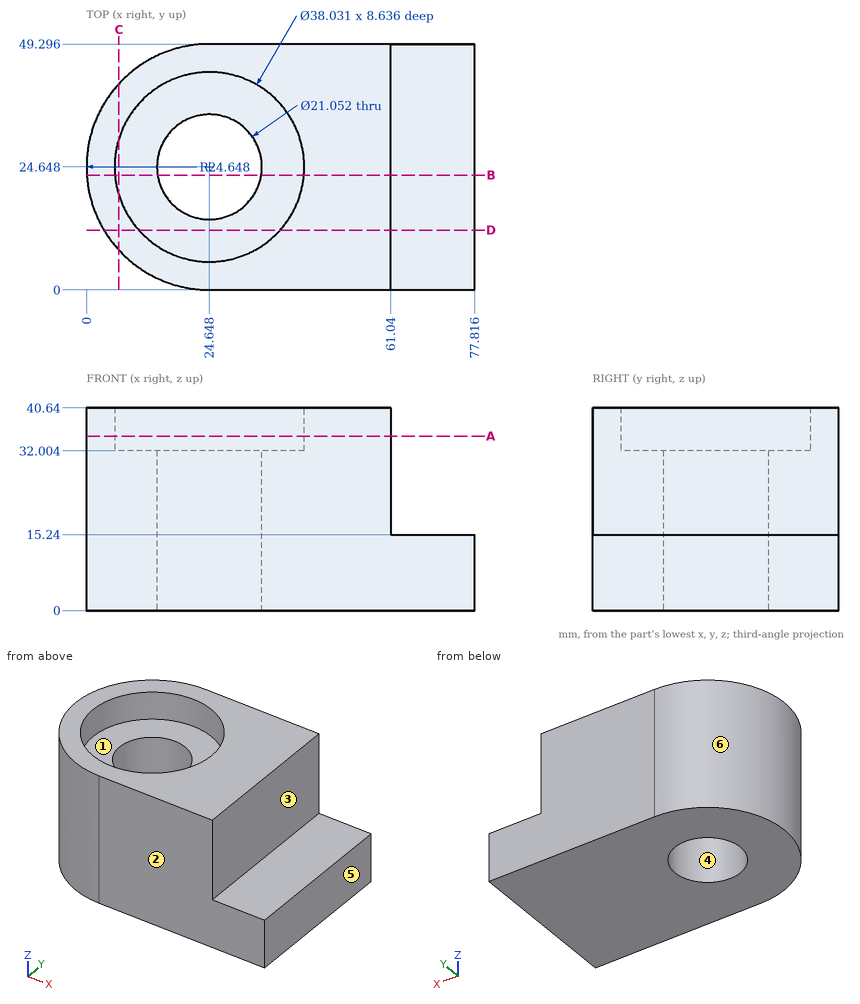
Source: three-view drawing plus pictorial views. Frame: mm from the lowest corner of the part. A direction names the side the tool comes from. Give positions to 0.01 mm unless a question says otherwise; leave off trailing zeros. Order: outer loops, then holes, each group sorted by start corner. A loop starts at its lowest first (then second) coordinate and runs counter-clockwise, first axis right, second up. Notation, with made-up numbers: M 0.25,-20.75 L 58.25,-20.75 A27 cw 58.25,7.25 Z; hole C 57.5,-27.75 d7. An arc over 180 degrees is marked long. One line per question, with ' | ' between items.
1) Access query for the marked faces 1, 2 and 3. Directions: +Z, -Z, +X, -X, +Y, -Y. A direction counts if a zero-diameter tool reaches every point of the face in a straight line with its end or side. Return the directions, or none.
Filled in:
face 1: +Z | face 2: +Z, -Z, +X, -X, -Y | face 3: +Z, +X, +Y, -Y
2) Ray query, L1, parallel to X at y = 17.5, z = 29 (1 decimal); L2, parallel to Y at x = 21.5, z = 36.5 (1 decimal); L3, parallel to Z at x = 34, y = 16.5. Return the intervals inside material, ascending.
Filled in:
L1: x = 1.1 to 16.9, 32.4 to 61 | L2: y = 0.2 to 5.9, 43.4 to 49.1 | L3: z = 0 to 32
3) Draft query along X for the marked faces 4, 5 and 6. Return one class per face: pulls with the +X half, pulls with the -X half, needs draft (parallel to the pull), parting line crosses it, or undercut.
Filled in:
face 4: undercut | face 5: pulls with the +X half | face 6: pulls with the -X half
4) Section B-B on y = 23. Output: boundary loops of the cut face in (x, z) (1 decimal), and give its area (3 significant figures).
Filled in:
outline: M 0.1,0 L 14.3,0 L 14.3,32 L 5.7,32 L 5.7,40.6 L 0.1,40.6 Z; M 35,0 L 77.8,0 L 77.8,15.2 L 61,15.2 L 61,40.6 L 43.6,40.6 L 43.6,32 L 35,32 Z | area: 1,740 mm2
5) Section D-D on y = 12. Output: boundary loops of the cut face in (x, z).
Filled in:
outline: M 3.49,0 L 77.82,0 L 77.82,15.24 L 61.04,15.24 L 61.04,40.64 L 38.85,40.64 L 38.85,32 L 10.45,32 L 10.45,40.64 L 3.49,40.64 Z
6) Section A-A on z = 35. Output: boundary loops of the cut face in (x, y) (1 decimal).
Filled in:
outline: M 24.6,0 L 61,0 L 61,49.3 L 24.6,49.3 A24.6 ccw Z; hole C 24.6,24.6 d38
7) Contact query for flat-ended pins moving along their axis: P1, Ø5, axis at x = 70.5, y = 25.5, coming from the +Z side; P2, Ø1, axis at x = 14.5, y = 16.5, coming from the +Z side; P3, Ø12, axis at y = 31, z = 26, coming from the -X side. Output: stop coordinate, or through.
Filled in:
P1: stops at z = 15.24 | P2: stops at z = 32 | P3: stops at x = 0
8) Section C-C on x = 6.5. Output: boundary loops of the cut face in (y, z).
Filled in:
outline: M 7.97,0 L 41.33,0 L 41.33,40.64 L 30.33,40.64 L 30.33,32 L 18.97,32 L 18.97,40.64 L 7.97,40.64 Z
